from build123d import *

# Parameters (mm, degrees)
SKETCH1_W           = 740
SKETCH1_H           = 1160
BOSS_EXTRUDE1_DEPTH = 5
FILLET1_R           = 10
CUT_EXTRUDE1_DEPTH  = 688.986191722
SKETCH3_W           = 360
SKETCH3_H           = 300
CUT_EXTRUDE2_DEPTH  = 688.986191722
FILLET2_R           = 100


with BuildPart() as part:
    # Sketch1 → Boss-Extrude1 (new body)
    with BuildSketch(Plane.XY):
        Rectangle(SKETCH1_W, SKETCH1_H)
    extrude(amount=BOSS_EXTRUDE1_DEPTH)

    # Fillet1
    fillet1_edges = [part.edges().sort_by_distance(p)[0] for p in [
        (370, -580, 2.5),
        (-370, -580, 2.5),
        (-370, 580, 2.5),
        (370, 580, 2.5),
    ]]
    fillet(fillet1_edges, radius=FILLET1_R)

    # Sketch2 → Cut-Extrude1 (cut, through all)
    with BuildSketch(Plane(origin=(0, 0, 0), x_dir=(-1, 0, 0), z_dir=(0, 0, -1))):
        Polygon((-370, -400), (120, 580), (-370, 580), align=None)
    extrude(amount=-CUT_EXTRUDE1_DEPTH, mode=Mode.SUBTRACT)

    # Sketch3 → Cut-Extrude2 (cut, through all)
    with BuildSketch(Plane.XY.offset(5)):
        with Locations((-370, 270)):
            Rectangle(SKETCH3_W, SKETCH3_H)
    extrude(amount=-CUT_EXTRUDE2_DEPTH, mode=Mode.SUBTRACT)

    # Fillet2
    fillet2_edges = [part.edges().sort_by_distance(p)[0] for p in [
        (-190, 120, 2.5),
        (-190, 420, 2.5),
    ]]
    fillet(fillet2_edges, radius=FILLET2_R)


solid = part.part
Here's how the part is built. I have some questions about the finished solid (model axes, mm). A direction names the side the tool comes from. Round coordinates to 2 decimals unless told otherwise and drop trailing zeros. Loops run counter-clockwise (first coordinate to the right, second up) from the corner with the lowest first, then second, coordinate; pieces in that order, holes last. Notation, with made-up numbers: (75, 84) - (112, 84) arc R18 cw to (112, 108) - close; hole circle Ø5 at (2.25, 52.25). An arc over 180 degrees is marked (long way). One line per question, with ' | ' between items. Start each with the question number.
Q1. Will this pin go through, and if not, where does the flat tip stop? pin 1 (2 mm diameter, centred on x = 255.5, z = 3, fed in from +Y).
Q2. I want a section at B-B (z = 2.55). Write out the boundary of the cut face in (x, y), then the cut area to 3 significant figures.
Q3. For faces 1 (the cylindrical face through (-218.516, 389.929, 2.465)), 2 (the flat face through (-87, -121, 5)), which set-ups out of +Z, -Z, +X, -X, +Y, -Y let a thin tool reach every point of the face, with its end or its side?
Q4. Please list where these lines run through material, in increasing order: line 1 (X direction, y = 76.5, z = 3.3); line 2 (X direction, y = -160.5, z = 4.3); line 3 (Y direction, x = 339.5, z = 2.45). Write a range as [from, to].
Q5. I want a section at A-A (x = -320). Write out the boundary of the cut face in (y, z).
Q6. I want a section at C-C (y = -13.5). Write out the boundary of the cut face in (x, z), then the cut area to 3 significant figures.
Q7. We'd pull the mould along Y, two halves only. Please class faces 3 (the flat face through (128.43, 83.14, 2.46)), 4 (the flat face through (-87, -121, 0)), 5 (the cylindrical face through (-220.071, 148.516, 2.465)): +Y half, -Y half, draft (parallel to the pull), parting line (faces both ways), or undercut.
Q8. I want a section at D-D (x = -9.5). Write out the boundary of the cut face in (y, z).
Response values:
1) pin 1: stops at y = -169
2) outline: (-370, -570) arc R10 ccw to (-360, -580) - (360, -580) arc R10 ccw to (370, -570) - (370, -400) - (-120, 580) - (-360, 580) arc R10 ccw to (-370, 570) - (-370, 420) - (-290, 420) arc R100 cw to (-190, 320) - (-190, 220) arc R100 cw to (-290, 120) - (-370, 120) - close | area: 569,000 mm²
3) face 1: +Z, -Z, -X | face 2: +Z, +X, -X, +Y, -Y
4) line 1: x = [-370, 131.75] | line 2: x = [-370, 250.25] | line 3: y = [-580, -339]
5) outline: (-580, 0) - (120, 0) - (120, 5) - (-580, 5) - close; (420, 0) - (580, 0) - (580, 5) - (420, 5) - close
6) outline: (-370, 0) - (176.75, 0) - (176.75, 5) - (-370, 5) - close | area: 2,730 mm²
7) face 3: +Y half | face 4: draft | face 5: undercut
8) outline: (-580, 0) - (359, 0) - (359, 5) - (-580, 5) - close
